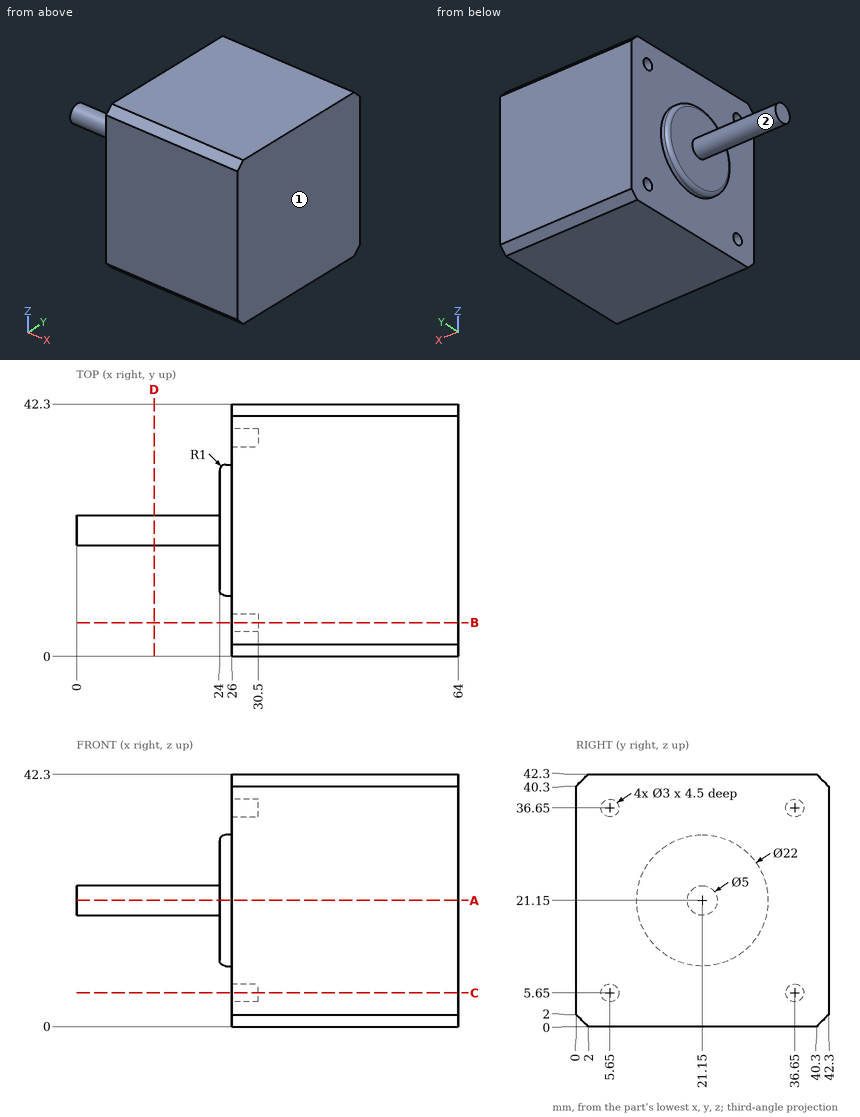
Source: three-view drawing plus pictorial views. Frame: mm from the lowest corner of the part. A direction names the side the tool comes from. Round coordinates to 2 decimals unless told otherwise and drop trailing zeros. Loops run counter-clockwise (first coordinate to the right, second up) from the corner with the lowest first, then second, coordinate; pieces in that order, holes last.
1. Contact query for flat-ended pins moving along their axis: pin 1 (0.9 mm diameter, centred on y = 5, z = 36, fed in from -X); pin 2 (3.5 mm diameter, centred on y = 5.5, z = 5.5, fed in from -X); pin 3 (12 mm diameter, centred on y = 15.5, z = 35, fed in from -X). Output: stop coordinate, or through.
2. Section query A-A on z = 21.15. Output: boundary loops of the cut face in (x, y).
3. Section query D-D on x = 13. Output: boundary loops of the cut face in (y, z).
4. Section query B-B on y = 5.65. Output: boundary loops of the cut face in (x, z), and give its area (3 significant figures).
5. Access query for the marked faces 1 and 2. Directions: +Z, -Z, +X, -X, +Y, -Y. A direction counts if a zero-diameter tool reaches every point of the face in a straight line with its end or side. Return the directions, or none.
6. Ray query, L1, parallel to Z at x = 27.05, y = 5.65; L2, parallel to Z at x = 29, y = 36. Return the intervals inside material, ascending.
Answers below:
1. pin 1: stops at x = 30.5
1. pin 2: stops at x = 26
1. pin 3: stops at x = 24
2. outline: (0, 18.65) - (24, 18.65) - (24, 11.15) arc R1 ccw to (25, 10.15) - (26, 10.15) - (26, 0) - (64, 0) - (64, 42.3) - (26, 42.3) - (26, 32.15) - (25, 32.15) arc R1 ccw to (24, 31.15) - (24, 23.65) - (0, 23.65) - close
3. outline: circle Ø5 at (21.15, 21.15)
4. outline: (26, 0) - (64, 0) - (64, 42.3) - (26, 42.3) - (26, 38.15) - (30.5, 38.15) - (30.5, 35.15) - (26, 35.15) - (26, 7.15) - (30.5, 7.15) - (30.5, 4.15) - (26, 4.15) - close
4. area: 1,580 mm2
5. face 1: +Z, -Z, +X, +Y, -Y
5. face 2: -X
6. L1: z = 0 to 4.15, 7.15 to 35.15, 38.15 to 42.3
6. L2: z = 0 to 4.3, 7 to 35.3, 38 to 42.3
